Build history of the part. All positions in model axes, mm. A direction names the side the tool comes from. Give positions to 0.01 mm unless a question says otherwise; leave off trailing zeros. Loops run counter-clockwise (first coordinate to the right, second up) from the corner with the lowest first, then second, coordinate; pieces in that order, holes last. Notation, with made-up numbers: (61.25, 2.25) - (108.25, 2.25) arc R7 ccw to (108.25, 12.25) - close; hole circle Ø9 at (15.25, 18). An arc over 180 degrees is marked (long way). Return JSON: item names as keys, results as strings. Group by question number.
1) Slice it at C-C (y = 1.15). List the corners of the cut face in (x, z).
2) 3-axis set-ups, long thin cutter, end or side, ignore diameter. For faces 1 (the face through (-13.145, 0.74, -6.432)), 2 (the face through (0, 1, -14)): which of +Z, -Z, +X, -X, +Y, -Y reach the whole face in a straight line?
3) Slice it at A-A (x = -1). List the corners of the cut face in (y, z), and give its area (3 significant figures).
4) Drill centre lines: probe 1 along X at (y, z) = (0.4, 0); probe 2 along Z at (x, y) = (1.5, 0.7); probe 3 along X at (y, z) = (1.15, -3). Where is each one in solid material? Low to high. Write a range as from..to.
5) Drop a flat-ended pin along its axis: pin 1 (4.5 mm diameter, centred on x = 21.15, z = 0, fed in from +Y). Give the stop position or say it passes through.
6) Slice it at D-D (z = 6.75). List the corners of the cut face in (x, y), and give its area (3 significant figures).
7) Slice it at B-B (z = 0). List the corners of the cut face in (x, y).
8) Mould opens along X. For faces 3 (the face through (12.145, 0.74, 6.764)), 4 (the face through (28, 1, 0)), 5 (the face through (0, 1, 14)) say: released by +X, released by -X, zero draft, split by the parting line, or undercut.
```python
from build123d import *

# Parameters (mm, degrees)
SKETCH1_R           = 2.5
BOSS_EXTRUDE1_DEPTH = 1.5


with BuildPart() as part:
    # Sketch1 → Boss-Extrude1 (new body)
    with BuildSketch(Plane(origin=(0, 0, 0), x_dir=(1, 0, 0), z_dir=(0, 1, 0))):
        Polygon((-13.5, 14), (13.5, 14), (28, 7.5), (28, -7.5), (13.5, -14), (-13.5, -14), (-28, -7.5), (-28, 7.5), align=None)
        with Locations((21.15, 0)):
            Circle(SKETCH1_R, mode=Mode.SUBTRACT)
        with Locations((-21.15, 0)):
            Circle(SKETCH1_R, mode=Mode.SUBTRACT)
        with BuildLine():
            Line((13, 4.333683406), (13, -4.666316594))
            ThreePointArc((13, -4.666316594), (12.121320344, -6.787636938), (10, -7.666316594))
            Line((10, -7.666316594), (-11, -7.666316594))
            ThreePointArc((-11, -7.666316594), (-13.121320344, -6.787636938), (-14, -4.666316594))
            Line((-14, -4.666316594), (-14, 4.333683406))
            ThreePointArc((-14, 4.333683406), (-13.121320344, 6.455003749), (-11, 7.333683406))
            Line((-11, 7.333683406), (10, 7.333683406))
            ThreePointArc((10, 7.333683406), (12.121320344, 6.455003749), (13, 4.333683406))
        make_face(mode=Mode.SUBTRACT)
    extrude(amount=BOSS_EXTRUDE1_DEPTH)


solid = part.part
```
Results:
{
 "1": {"outline": "(-28, -7.5) - (-13.5, -14) - (13.5, -14) - (28, -7.5) - (28, 7.5) - (13.5, 14) - (-13.5, 14) - (-28, 7.5) - close; hole circle Ø5 at (-21.15, 0); hole (-14, -4.33) arc R3 ccw to (-11, -7.33) - (10, -7.33) arc R3 ccw to (13, -4.33) - (13, 4.67) arc R3 ccw to (10, 7.67) - (-11, 7.67) arc R3 ccw to (-14, 4.67) - close; hole circle Ø5 at (21.15, 0)"},
 "2": {"face 1": "+Y, -Y", "face 2": "-Z, +X, -X, +Y, -Y"},
 "3": {"outline": "(0, -14) - (1.5, -14) - (1.5, -7.33) - (0, -7.33) - close; (0, 7.67) - (1.5, 7.67) - (1.5, 14) - (0, 14) - close", "area": "19.5 mm2"},
 "4": {"probe 1": "-28..-23.65, -18.65..-14, 13..18.65, 23.65..28", "probe 2": "-14..-7.33, 7.67..14", "probe 3": "-28..-14, 13..28"},
 "5": {"pin 1": "through"},
 "6": {"outline": "(-28, 0) - (-13.16, 0) - (-13.16, 1.5) - (-28, 1.5) - close; (12.16, 0) - (28, 0) - (28, 1.5) - (12.16, 1.5) - close", "area": "46.0 mm2"},
 "7": {"outline": "(-28, 0) - (-23.65, 0) - (-23.65, 1.5) - (-28, 1.5) - close; (-18.65, 0) - (-14, 0) - (-14, 1.5) - (-18.65, 1.5) - close; (13, 0) - (18.65, 0) - (18.65, 1.5) - (13, 1.5) - close; (23.65, 0) - (28, 0) - (28, 1.5) - (23.65, 1.5) - close"},
 "8": {"face 3": "undercut", "face 4": "released by +X", "face 5": "zero draft"}
}
